Can you work these out from the model? Positions are in its coordinate system, mm. Face numbers are marked on the shaded views. A direction names the side the tool comes from. Give positions to 0.01 mm unless a question says otherwise; leave off trailing zeros. Loops run counter-clockwise (first coordinate to the right, second up) from the corner with the lowest first, then second, coordinate; pieces in that order, holes last. Notation, with made-up numbers: (72, -36.5) - (115, -36.5) arc R27 cw to (115, -10.5) - close; hole circle Ø9 at (43, -15). An arc over 180 degrees is marked (long way). Answer as a JSON object with one key per item and string values. Group by question number.
Item 1: Which directions (+Z, -Z, +X, -X, +Y, -Y) give clear straight access to the entire face, cutting with the end or side of a thin tool? Please do the marked faces 4 and 5.
Item 2: Thinking about a two-plate mould opening in X: for the marked faces 1, 2 and 3, which applies, pulls with the +X half, pulls with the -X half, needs draft (parallel to the pull), parting line crosses it, or undercut?
Item 3: Suppose I cut it at A-A on z = -1.5. Write out the boundary of the cut face in (x, y), and give its area (3 significant figures).
Item 4: Will these pins go through, and if not, where does the flat tip stop? pin 1 (2 mm diameter, centred on y = 1.5, z = -12, fed in from -X); pin 2 (3 mm diameter, centred on x = -0.5, y = -1, fed in from +Z); pin 3 (4 mm diameter, centred on y = -3, z = -8.5, fed in from +X); pin 4 (1 mm diameter, centred on y = 1, z = -5.5, fed in from +X).
Item 5: Please list where these lines run through material, in increasing order: L1, parallel to Z at x = -1.5, y = 1; L2, parallel to X at y = 1.75, z = 2; L3, parallel to Y at x = 1, z = -9.5.
from build123d import *

# Parameters (mm, degrees)
ENL_V_MAT_EXTRU_1_DEPTH = 1.7


with BuildPart() as part:
    # Esquisse1 → Révolution1 (revolve)
    with BuildSketch(Plane(origin=(0, 0, 0), x_dir=(0, 0, -1), z_dir=(1, 0, 0))):
        with BuildLine():
            Line((-3.1, 0), (-3.1, 2))
            ThreePointArc((-3.1, 2), (-2.617577029, 3.312440475), (-1.4, 4))
            Line((-1.4, 4), (0, 4))
            Line((0, 4), (0, 2))
            Line((0, 2), (16, 2))
            Line((16, 2), (16, 0))
            Line((16, 0), (-3.1, 0))
        make_face()
    revolve(axis=Axis((0, 0, 3.1), (0, 0, 1)))

    # Esquisse2 → Enlèv. mat.-Extru.1 (cut)
    with BuildSketch(Plane.XY.offset(3.1)):
        with BuildLine():
            ThreePointArc((-0.343897346, 1.728888708), (0, 2), (0.343897346, 1.728888708))
            ThreePointArc((0.343897346, 1.728888708), (0.712882715, 1.234749083), (1.325312868, 1.162268192))
            ThreePointArc((1.325312868, 1.162268192), (1.732050808, 1), (1.669210214, 0.566620516))
            ThreePointArc((1.669210214, 0.566620516), (1.42576543, 0), (1.669210214, -0.566620516))
            ThreePointArc((1.669210214, -0.566620516), (1.732050808, -1), (1.325312868, -1.162268192))
            ThreePointArc((1.325312868, -1.162268192), (0.712882715, -1.234749083), (0.343897346, -1.728888708))
            ThreePointArc((0.343897346, -1.728888708), (0, -2), (-0.343897346, -1.728888708))
            ThreePointArc((-0.343897346, -1.728888708), (-0.712882715, -1.234749083), (-1.325312868, -1.162268192))
            ThreePointArc((-1.325312868, -1.162268192), (-1.732050808, -1), (-1.669210214, -0.566620516))
            ThreePointArc((-1.669210214, -0.566620516), (-1.42576543, 0), (-1.669210214, 0.566620516))
            ThreePointArc((-1.669210214, 0.566620516), (-1.732050808, 1), (-1.325312868, 1.162268192))
            ThreePointArc((-1.325312868, 1.162268192), (-0.712882715, 1.234749083), (-0.343897346, 1.728888708))
        make_face()
    extrude(amount=-ENL_V_MAT_EXTRU_1_DEPTH, mode=Mode.SUBTRACT)


solid = part.part
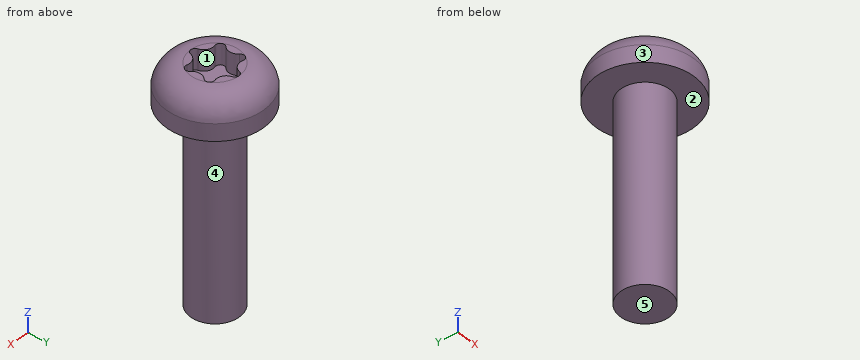
Worked out:
{
 "1": {"face 4": "-Z", "face 5": "-Z, +X, -X, +Y, -Y"},
 "2": {"face 1": "undercut", "face 2": "needs draft", "face 3": "parting line crosses it"},
 "3": {"outline": "circle Ø4 at (0, 0)", "area": "12.6 mm2"},
 "4": {"pin 1": "stops at x = -1.94", "pin 2": "stops at z = 3.1", "pin 3": "stops at x = 1.73", "pin 4": "stops at x = 1.94"},
 "5": {"L1": "z = -16 to 1.4", "L2": "x = -3.38 to -0.34, 0.34 to 3.38", "L3": "y = -1.73 to 1.73"}
}
